CAD build for the part. Positions are in the model's coordinates, mm. Face numbers are marked on the shaded views. A direction names the side the tool comes from. Coordinates: 2 decimals unless noted, no trailing zeros. Loops run counter-clockwise (first coordinate to the right, second up) from the corner with the lowest first, then second, coordinate; pieces in that order, holes last. Notation, with made-up numbers: (86, -35.5) -> (118, -35.5) arc R16 cw to (118, -18.5) -> close; hole circle Ø6 at (43, 53). An arc over 180 degrees is marked (long way). Write item = value, one per line. Start each with the question number.
(1) Tool access for the marked faces 1, 2, 3, 4 and 5: list every direction of +Z, -Z, +X, -X, +Y, -Y with a clear straight run to the whole face (end or side of a thin tool).
(2) Drill centre lines: line 1 (Y direction, x = 2.44, z = 1.7); line 2 (X direction, y = 2.55, z = 1.2); line 3 (X direction, y = 2.55, z = 0.85). Where is each one in solid material? Low to high. Write a range as from..to.
(3) Band-saw the part on D-D (x = 5.5). Write the cut outline in (y, z).
(4) Pull direction Z, two halves, no side cores. Call the marked faces 6, 7 and 8: +Z half, -Z half, draft (parallel to the pull), parting line (faces both ways), or undercut.
(5) Flat gauge pins, fed straight in: P1, Ø2.5, axis at x = 2.44, y = 2.55, coming from the +Z side; P2, Ø3, axis at x = 23.5, z = 1, coming from the -Y side; P3, Ø5, axis at x = 9, y = 4, coming from the +Z side; P4, Ø1, axis at x = 6.5, z = 5, coming from the -Y side. Where does each tip first touch, or does it go through?
(6) Band-saw the part on A-A (x = 2.44). Write the cut outline in (y, z), and give its area (3 significant figures).
(7) Band-saw the part on C-C (z = 2). Count the separate pieces of the cut face and the enclosed holes in it, and give its area (3 significant figures).
```python
from build123d import *

# Parameters (mm, degrees)
SKETCH1_W           = 26.99
SKETCH1_H           = 10
SKETCH1_R           = 0.96
BOSS_EXTRUDE1_DEPTH = 5
SKETCH3_R           = 4
BOSS_EXTRUDE2_DEPTH = 4.75
FILLET1_R           = 2
FILLET2_R           = 2
CHAMFER1_SIZE       = 0.8
SKETCH6_W           = 3.842122027
SKETCH6_H           = 10
CUT_EXTRUDE1_DEPTH  = 41
CHAMFER3_START      = 10.25
CHAMFER3_DEPTH      = 9.5
SKETCH7_W           = 13.45
SKETCH7_H           = 4.563034457
CUT_EXTRUDE2_DEPTH  = 1
CHAMFER5_SIZE       = 1


with BuildPart() as part:
    # Sketch1 → Boss-Extrude1 (new body)
    with BuildSketch(Plane.XY):
        with Locations((13.495, 5)):
            Rectangle(SKETCH1_W, SKETCH1_H)
        with Locations((2.44, 2.55)):
            Circle(SKETCH1_R, mode=Mode.SUBTRACT)
        with Locations((24.99, 2.55)):
            Circle(SKETCH1_R, mode=Mode.SUBTRACT)
    extrude(amount=BOSS_EXTRUDE1_DEPTH)

    # Sketch3 → Boss-Extrude2 (add, symmetric)
    with BuildSketch(Plane.ZY.offset(-15)):
        with Locations((2.568998912, -3.622468738)):
            Circle(SKETCH3_R)
        Polygon((0.512453731, -3.622468738), (1.114801869, -5.076665781), (2.568998912, -5.679013919), (4.023195955, -5.076665781), (4.625544092, -3.622468738), (4.023195955, -2.168271695), (2.568998912, -1.565923558), (1.114801869, -2.168271695), align=None, mode=Mode.SUBTRACT)
    extrude(amount=BOSS_EXTRUDE2_DEPTH, both=True)

    # Fillet1
    # the kernel refuses this fillet: 2 mm, written as the material it adds along each edge
    with BuildSketch(Plane(origin=(19.75, 0, 0.872614451), x_dir=(0, 0, -1), z_dir=(-1, 0, 0))) as fillet1_piece_1:
        with BuildLine():
            CenterArc((2.851261839, -0.291469576), FILLET1_R, 139.283020083, 32.337148469)
            ThreePointArc((1.335379739, 1.013176529), (0.721358104, 0.435852839), (0, 0))
            Line((0, 0), (0.872614451, 0))
        make_face()
    extrude(amount=9.5)
    with BuildSketch(Plane(origin=(19.75, 0, 4.265383373), x_dir=(0, 0, 1), z_dir=(-1, 0, 0))) as fillet1_piece_2:
        with BuildLine():
            CenterArc((2.674069858, 0.488386288), FILLET1_R, 194.13415607, 29.112659272)
            ThreePointArc((1.217251752, -0.881898721), (0.650423795, -0.383257259), (0, 0))
            Line((0, 0), (0.734616627, 0))
        make_face()
    extrude(amount=9.5)

    # Fillet2
    # the kernel refuses this fillet: 2 mm, written as the material it adds along each edge
    with BuildSketch(Plane(origin=(19.75, 0, 0), x_dir=(0, 1, 0), z_dir=(-1, 0, 0))) as fillet2_piece_1:
        with BuildLine():
            CenterArc((0.266521997, 2), FILLET2_R, 229.596597584, 40.403402416)
            Line((-1.029808248, 0.477000363), (-1.159441272, 0.324700399))
            ThreePointArc((-1.159441272, 0.324700399), (-1.143641139, 0.311177078), (-0.029146958, -0.197864739))
            Line((-0.029146958, -0.197864739), (0, -0.2))
            Line((0, -0.2), (0.266521997, -0.2))
            Line((0.266521997, -0.2), (0.266521997, 0))
        make_face()
    extrude(amount=9.5)
    with BuildSketch(Plane(origin=(19.75, 0, 5), x_dir=(0, -0.870596677984774, 0.491997382393317), z_dir=(-1, 0, 0))) as fillet2_piece_2:
        with BuildLine():
            CenterArc((0.615688034, 1.949333304), FILLET2_R, 240.528051524, 42.396189725)
            Line((-0.368306731, 0.208139948), (-0.466706207, 0.034020613))
            Line((-0.466706207, 0.034020613), (-0.098399476, -0.174119336))
            Line((-0.098399476, -0.174119336), (-0.052901843, -0.192876631))
            ThreePointArc((-0.052901843, -0.192876631), (1.052854803, -0.20795909), (1.10774555, -0.19493333))
            Line((1.10774555, -0.19493333), (1.063013048, 0))
        make_face()
    extrude(amount=9.5)

    # Chamfer1
    # the kernel refuses this chamfer: 0.8 mm, written as the material it takes off along each edge
    with BuildSketch(Plane(origin=(19.75, 0.266521997, -2), x_dir=(0, -0.648165122631187, 0.7614998186503384), z_dir=(0, -0.7614998186503384, -0.648165122631187))) as chamfer1_piece_1_section:
        Polygon((2, CHAMFER1_SIZE), (2 + CHAMFER1_SIZE, 0), (2, 0), align=None)
    chamfer1_piece_1 = revolve(axis=Axis((19.75, 0.266521997, -2), (-1, 0, 0)), revolution_arc=99.346805501, mode=Mode.PRIVATE)
    chamfer1_piece_1 = split(chamfer1_piece_1, bisect_by=Plane(origin=(19.75, 0, -2), z_dir=(0, -1, 0)), keep=Keep.TOP, mode=Mode.PRIVATE)
    add(chamfer1_piece_1, mode=Mode.SUBTRACT)
    with BuildSketch(Plane(origin=(19.75, 0.266521997, -2), x_dir=(0, -0.648165122631187, 0.7614998186503384), z_dir=(0, -0.7614998186503384, -0.648165122631187))) as chamfer1_piece_2_section:
        Polygon((2, CHAMFER1_SIZE), (2 + CHAMFER1_SIZE, 0), (2, 0), align=None)
    chamfer1_piece_2 = revolve(axis=Axis((19.75, 0.266521997, -2), (-1, 0, 0)), revolution_arc=99.346805501, mode=Mode.PRIVATE)
    chamfer1_piece_2 = split(chamfer1_piece_2, bisect_by=Plane(origin=(19.75, 0.266521997, 0), z_dir=(0, 0, -1)), keep=Keep.TOP, mode=Mode.PRIVATE)
    add(chamfer1_piece_2, mode=Mode.SUBTRACT)
    with BuildSketch(Plane(origin=(19.75, 0.423050926, 7), x_dir=(0, 0.8566624684959867, -0.515877325602088), z_dir=(0, 0.515877325602088, 0.8566624684959867))) as chamfer1_piece_3_section:
        Polygon((2, CHAMFER1_SIZE), (2 + CHAMFER1_SIZE, 0), (2, 0), align=None)
    chamfer1_piece_3 = revolve(axis=Axis((19.75, 0.423050926, 7), (-1, 0, 0)), revolution_arc=101.340075028, mode=Mode.PRIVATE)
    chamfer1_piece_3 = split(chamfer1_piece_3, bisect_by=Plane(origin=(19.75, 0, 7), z_dir=(0, -1, 0)), keep=Keep.TOP, mode=Mode.PRIVATE)
    add(chamfer1_piece_3, mode=Mode.SUBTRACT)
    with BuildSketch(Plane(origin=(19.75, 0.423050926, 7), x_dir=(0, 0.8566624684959867, -0.515877325602088), z_dir=(0, 0.515877325602088, 0.8566624684959867))) as chamfer1_piece_4_section:
        Polygon((2, CHAMFER1_SIZE), (2 + CHAMFER1_SIZE, 0), (2, 0), align=None)
    chamfer1_piece_4 = revolve(axis=Axis((19.75, 0.423050926, 7), (-1, 0, 0)), revolution_arc=101.340075028, mode=Mode.PRIVATE)
    chamfer1_piece_4 = split(chamfer1_piece_4, bisect_by=Plane(origin=(19.75, 0.423050926, 5), z_dir=(0, 0, 1)), keep=Keep.TOP, mode=Mode.PRIVATE)
    add(chamfer1_piece_4, mode=Mode.SUBTRACT)
    with BuildSketch(Plane(origin=(19.75, -3.622468738, 2.568998912), x_dir=(0, 0.6742532774459821, 0.7385001813495726), z_dir=(0, 0.7385001813495726, -0.6742532774459821))) as chamfer1_piece_5:
        Polygon((4 - CHAMFER1_SIZE, 0), (4, -CHAMFER1_SIZE), (4, 0), align=None)
    revolve(axis=Axis((19.75, -3.622468738, 2.568998912), (1, 0, 0)), revolution_arc=262.799592141, mode=Mode.SUBTRACT)
    with BuildSketch(Plane(origin=(10.25, 0.266521997, -2), x_dir=(0, -0.648165122631187, 0.7614998186503384), z_dir=(0, -0.7614998186503384, -0.648165122631187))) as chamfer1_piece_6_section:
        Polygon((2 + CHAMFER1_SIZE, 0), (2, -CHAMFER1_SIZE), (2, 0), align=None)
    chamfer1_piece_6 = revolve(axis=Axis((10.25, 0.266521997, -2), (-1, 0, 0)), revolution_arc=99.346805501, mode=Mode.PRIVATE)
    chamfer1_piece_6 = split(chamfer1_piece_6, bisect_by=Plane(origin=(10.25, 0, -2), z_dir=(0, -1, 0)), keep=Keep.TOP, mode=Mode.PRIVATE)
    add(chamfer1_piece_6, mode=Mode.SUBTRACT)
    with BuildSketch(Plane(origin=(10.25, 0.266521997, -2), x_dir=(0, -0.648165122631187, 0.7614998186503384), z_dir=(0, -0.7614998186503384, -0.648165122631187))) as chamfer1_piece_7_section:
        Polygon((2 + CHAMFER1_SIZE, 0), (2, -CHAMFER1_SIZE), (2, 0), align=None)
    chamfer1_piece_7 = revolve(axis=Axis((10.25, 0.266521997, -2), (-1, 0, 0)), revolution_arc=99.346805501, mode=Mode.PRIVATE)
    chamfer1_piece_7 = split(chamfer1_piece_7, bisect_by=Plane(origin=(10.25, 0.266521997, 0), z_dir=(0, 0, -1)), keep=Keep.TOP, mode=Mode.PRIVATE)
    add(chamfer1_piece_7, mode=Mode.SUBTRACT)
    with BuildSketch(Plane(origin=(10.25, 0.423050926, 7), x_dir=(0, 0.8566624684959867, -0.515877325602088), z_dir=(0, 0.515877325602088, 0.8566624684959867))) as chamfer1_piece_8_section:
        Polygon((2, -CHAMFER1_SIZE), (2 + CHAMFER1_SIZE, 0), (2, 0), align=None)
    chamfer1_piece_8 = revolve(axis=Axis((10.25, 0.423050926, 7), (-1, 0, 0)), revolution_arc=101.340075028, mode=Mode.PRIVATE)
    chamfer1_piece_8 = split(chamfer1_piece_8, bisect_by=Plane(origin=(10.25, 0, 7), z_dir=(0, -1, 0)), keep=Keep.TOP, mode=Mode.PRIVATE)
    add(chamfer1_piece_8, mode=Mode.SUBTRACT)
    with BuildSketch(Plane(origin=(10.25, 0.423050926, 7), x_dir=(0, 0.8566624684959867, -0.515877325602088), z_dir=(0, 0.515877325602088, 0.8566624684959867))) as chamfer1_piece_9_section:
        Polygon((2, -CHAMFER1_SIZE), (2 + CHAMFER1_SIZE, 0), (2, 0), align=None)
    chamfer1_piece_9 = revolve(axis=Axis((10.25, 0.423050926, 7), (-1, 0, 0)), revolution_arc=101.340075028, mode=Mode.PRIVATE)
    chamfer1_piece_9 = split(chamfer1_piece_9, bisect_by=Plane(origin=(10.25, 0.423050926, 5), z_dir=(0, 0, 1)), keep=Keep.TOP, mode=Mode.PRIVATE)
    add(chamfer1_piece_9, mode=Mode.SUBTRACT)
    with BuildSketch(Plane(origin=(10.25, -3.622468738, 2.568998912), x_dir=(0, 0.6742532774459821, 0.7385001813495726), z_dir=(0, 0.7385001813495726, -0.6742532774459821))) as chamfer1_piece_10:
        Polygon((4 - CHAMFER1_SIZE, 0), (4, CHAMFER1_SIZE), (4, 0), align=None)
    revolve(axis=Axis((10.25, -3.622468738, 2.568998912), (1, 0, 0)), revolution_arc=262.799592141, mode=Mode.SUBTRACT)

    # Sketch6 → Cut-Extrude1 (cut)
    with BuildSketch(Plane(origin=(0, 0, 0), x_dir=(0, 0, -1), z_dir=(1, 0, 0))):
        with Locations((-4.430776166, 5)):
            Rectangle(SKETCH6_W, SKETCH6_H)
    extrude(amount=CUT_EXTRUDE1_DEPTH, mode=Mode.SUBTRACT)

    # Chamfer3: read off the stored shape, not the designer's step
    # Chamfer3 outline → Chamfer3 (add)
    with BuildSketch(Plane.YZ.offset(CHAMFER3_START)):
        with BuildLine():
            ThreePointArc((0.507913909, 5.001801243), (0.252566824, 5.007279455), (0, 5.045255026))
            Line((0, 5.045255026), (0, 2.509715152))
            Line((0, 2.509715152), (3, 2.509715152))
            Line((3, 2.509715152), (0.507913909, 5.001801243))
        make_face()
    extrude(amount=CHAMFER3_DEPTH)

    # Chamfer3 2 outline → Chamfer3 2 (revolve, cut)
    with BuildSketch(Plane(origin=(0, 0.423050926, 7), x_dir=(0, 1, 0), z_dir=(0, 0, -1))):
        Polygon((2, 19.75), (2, 18.95), (2.8, 19.75), align=None)
        Polygon((2.8, 10.25), (2, 11.05), (2, 10.25), align=None)
    revolve(axis=Axis((0, 0.423050926, 7), (1, 0, 0)), mode=Mode.SUBTRACT)

    # Sketch7 → Cut-Extrude2 (cut)
    with BuildSketch(Plane(origin=(0, 0, 0), x_dir=(-1, 0, 0), z_dir=(0, 0, -1))):
        with Locations((-13.715, 3.718482772)):
            Rectangle(SKETCH7_W, SKETCH7_H)
    extrude(amount=-CUT_EXTRUDE2_DEPTH, mode=Mode.SUBTRACT)

    # Chamfer5
    chamfer5_edges = [part.edges().sort_by_distance(p)[0] for p in [
        (13.715, 6, 1),
        (6.99, 3.718482772, 1),
        (13.715, 1.436965543, 1),
        (20.44, 3.718482772, 1),
    ]]
    chamfer(chamfer5_edges, length=CHAMFER5_SIZE - 0.0001)  # a hair under: the kernel refuses the full size


solid = part.part
```
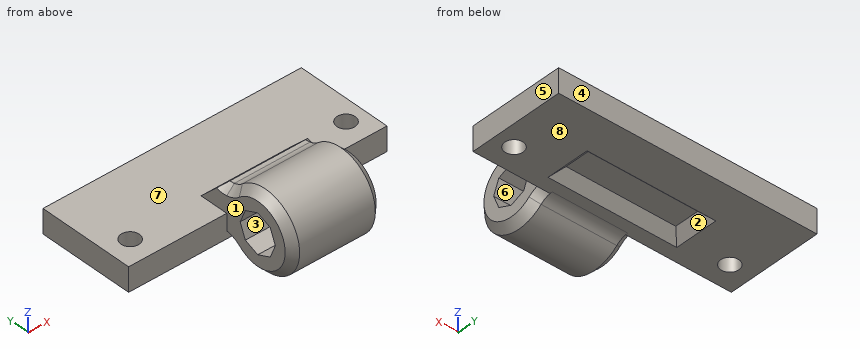
Findings below:
q1.face_1 = +Z, -X, -Y
q1.face_2 = -Z
q1.face_3 = +X, -X
q1.face_4 = +Z, -Z, +X, -X, +Y
q1.face_5 = +Z, -Z, +X, +Y, -Y
q2.line_1 = 0..1.59, 3.51..10
q2.line_2 = 0..1.48, 3.4..24.03, 25.95..26.99
q2.line_3 = 0..1.48, 3.4..7.84, 19.59..24.03, 25.95..26.99
q3.outline = (0, 0) -> (10, 0) -> (10, 2.51) -> (0, 2.51) -> close
q4.face_6 = undercut
q4.face_7 = +Z half
q4.face_8 = -Z half
q5.P1 = 2.51
q5.P2 = 0
q5.P3 = 3.67
q5.P4 = through
q6.outline = (0, 0) -> (1.59, 0) -> (1.59, 2.51) -> (0, 2.51) -> close; (3.51, 0) -> (10, 0) -> (10, 2.51) -> (3.51, 2.51) -> close
q6.area = 20.3 mm²
q7.separate_pieces = 2
q7.enclosed_holes = 2
q7.area = 301 mm²
